The model under review builds one solid part; all positions refer to its coordinate system, in mm. A direction names the side the tool comes from. Round coordinates to 2 decimals unless told otherwise and drop trailing zeros. Order: outer loops, then holes, each group sorted by start corner. A loop starts at its lowest first (then second) coordinate and runs counter-clockwise, first axis right, second up. Notation, with made-up numbers: M -6,-28.5 L 40,-28.5 A34 ccw 40,4.5 Z; hole C 40,59 d10. An arc over 180 degrees is marked long. Answer as CSV lines item,"result". Start each with the question number.
from build123d import *

# Parameters (mm, degrees)
ESQUISSE1_W        = 80
ESQUISSE1_H        = 49.6
BOSS_EXTRU_1_DEPTH = 30
COQUE1_T           = -0.8
CONG_1_R           = 1.6


with BuildPart() as part:
    # Esquisse1 → Boss.-Extru.1 (new body)
    with BuildSketch(Plane.XY):
        Rectangle(ESQUISSE1_W, ESQUISSE1_H)
    extrude(amount=BOSS_EXTRU_1_DEPTH)

    # Coque1
    coque1_openings = [part.faces().sort_by_distance(p)[0] for p in [
        (0, 0, 30),
    ]]
    offset(amount=COQUE1_T, openings=coque1_openings, kind=Kind.INTERSECTION)

    # Congé1
    cong_1_edges = [part.edges().sort_by_distance(p)[0] for p in [
        (39.2, 0, 0.8),
        (39.2, -24, 15.4),
        (0, 24, 0.8),
        (39.2, 24, 15.4),
        (-39.2, 0, 0.8),
        (-39.2, 24, 15.4),
        (0, -24, 0.8),
        (-39.2, -24, 15.4),
        (40, -24.8, 15),
        (-40, -24.8, 15),
        (-40, 24.8, 15),
        (40, 24.8, 15),
    ]]
    fillet(cong_1_edges, radius=CONG_1_R)


solid = part.part
Item 1: Tool access review of faces 1 (the cylindrical face through (38.74, 0.31, 1.28)), 2 (the cylindrical face through (-39.54, 24.32, 15.21)): name each direction out of +Z, -Z, +X, -X, +Y, -Y from which nothing blocks a thin tool from reaching the whole face with its end or side.
Item 2: Wall thickness on probe 1 along Y at (x, z) = (16, 17); probe 2 along X at (y, z) = (-2, 3.75); probe 3 along Z at (x, y) = (5.5, -12): over which ranges is each line inside the solid? List them lowest first. Write a range as [from, to].
Item 3: Consider section A-A (x = 0). State the section outline as (y, z) points, and give its area (3 significant figures).
Item 4: For pin 1 (3 mm diameter, centred on x = 12, y = 18.5, fed in from +Z), flat-tipped, find the tip position at first contact; note if it passes through.
Item 5: The part is to be moulded in two halves that separate along Y. For faces 3 (the flat face through (-1, 0, 0)), 4 (the cylindrical face through (39.52, -24.34, 15.21)), 5 (the flat face through (-1, 24.8, 15)), 6 (the cylindrical face through (38.72, -23.54, 16.39)), say which applies: +Y half, -Y half, draft (parallel to the pull), parting line (faces both ways), or undercut.
Item 6: Consider section B-B (z = 21.75). State the section outline as (x, y) points, and give its area (3 significant figures).
Item 7: Consider section C-C (y = -14.5). State the section outline as (x, z) points, and give its area (3 significant figures).
Reported:
1,face 1,"+Z"
1,face 2,"+Z, -Z, -X, +Y"
2,probe 1,"y = [-24.8, -24], [24, 24.8]"
2,probe 2,"x = [-40, -39.2], [39.2, 40]"
2,probe 3,"z = [0, 0.8]"
3,outline,"M -24.8,0 L 24.8,0 L 24.8,30 L 24,30 L 24,2.4 A1.6 cw 22.4,0.8 L -22.4,0.8 A1.6 cw -24,2.4 L -24,30 L -24.8,30 Z"
3,area,"87.5 mm²"
4,pin 1,"stops at z = 0.8"
5,face 3,"draft"
5,face 4,"-Y half"
5,face 5,"+Y half"
5,face 6,"undercut"
6,outline,"M -40,-23.2 A1.6 ccw -38.4,-24.8 L 38.4,-24.8 A1.6 ccw 40,-23.2 L 40,23.2 A1.6 ccw 38.4,24.8 L -38.4,24.8 A1.6 ccw -40,23.2 Z; hole M -39.2,-22.4 A1.6 ccw -37.6,-24 L 37.6,-24 A1.6 ccw 39.2,-22.4 L 39.2,22.4 A1.6 ccw 37.6,24 L -37.6,24 A1.6 ccw -39.2,22.4 Z"
6,area,"205 mm²"
7,outline,"M -40,0 L 40,0 L 40,30 L 39.2,30 L 39.2,2.4 A1.6 cw 37.6,0.8 L -37.6,0.8 A1.6 cw -39.2,2.4 L -39.2,30 L -40,30 Z"
7,area,"112 mm²"
